Input: part model. Units: mm. Frame: model coordinates. A direction names the side the tool comes from. Coordinates: 2 decimals unless noted, no trailing zeros. Loops run counter-clockwise (first coordinate to the right, second up) from the corner with the lowest first, then second, coordinate; pieces in that order, holes last. Notation, with made-up numbers: (72, 79.5) -> (93, 79.5) arc R16 cw to (93, 110.5) -> close; hole circle Ø1 at (28.5, 53.25). An arc over 180 degrees is marked (long way). Answer as a JSON object with one key per item and string values.
Autodesk Inventor part; units mm, degrees
ref_plane "YZ Plane" through (0, 0, 0) normal (1, 0, 0) x (0, 1, 0)
ref_plane "XZ Plane" through (0, 0, 0) normal (0, 1, 0) x (-1, 0, 0)
ref_plane "XY Plane" through (0, 0, 0) normal (0, 0, 1) x (1, 0, 0)
sketch "Sketch1" plane through (0, 0, 0) normal (0, 0, 1) x (1, 0, 0)
  circle A0 centre (0, 0) radius 31.75
  circle A1 centre (0, 0) radius 25.4
  circle A2 centre (0, 0) radius 6.35
  dimension "d0" = 63.5
  dimension "d1" = 50.8
  dimension "d2" = 12.7
extrude "Extrusion1" add sketch "Sketch1" along normal blind 6.35 contours A0
extrude "Extrusion2" add sketch "Sketch1" along normal blind 6.35 contours A1
extrude "Extrusion3" add sketch "Sketch1" against normal blind 19.05 contours A1
properties part number "2.5ingear proxy"
1. Pin query (flat end, axial travel): P1, Ø1.5, axis at y = -15.5, z = -12, coming from the +X side; P2, Ø1, axis at x = -3.5, z = -1, coming from the +Y side; P3, Ø12, axis at y = 6.5, z = -9, coming from the -X side. Return the tip coordinate at first contact, or that it passes through.
Reply:
{"P1": "stops at x = 20.68", "P2": "stops at y = 25.22", "P3": "stops at x = -25.4"}
2. Section query D-D (x = 13). Return loops of the section in (y, z), plus the area to 3 significant figures.
Reply:
{"outline": "(-28.97, 0) -> (-21.82, 0) -> (-21.82, -19.05) -> (21.82, -19.05) -> (21.82, 0) -> (28.97, 0) -> (28.97, 6.35) -> (-28.97, 6.35) -> close", "area": "1,200 mm2"}
3. Section query A-A (x = 0). Return loops of the section in (y, z).
Reply:
{"outline": "(-31.75, 0) -> (-25.4, 0) -> (-25.4, -19.05) -> (-6.35, -19.05) -> (-6.35, 6.35) -> (-31.75, 6.35) -> close; (6.35, -19.05) -> (25.4, -19.05) -> (25.4, 0) -> (31.75, 0) -> (31.75, 6.35) -> (6.35, 6.35) -> close"}
4. Access query for faces 1 (the face through (-14.3, 21.3, 0)), 2 (the face through (7, 0, 6.35)). Directions: +Z, -Z, +X, -X, +Y, -Y. A direction counts if a zero-diameter tool reaches every point of the face in a straight line with its end or side. Return the directions, or none.
Reply:
{"face 1": "-Z", "face 2": "+Z, +X, -X, +Y, -Y"}
5. Section query C-C (y = 22). Return loops of the section in (x, z).
Reply:
{"outline": "(-22.89, 0) -> (-12.69, 0) -> (-12.69, -19.05) -> (12.69, -19.05) -> (12.69, 0) -> (22.89, 0) -> (22.89, 6.35) -> (-22.89, 6.35) -> close"}
6. Mould query, pull axis Y, two halves, no side actions, for faces 3 (the face through (-5.506, -24.796, -9.392)), 4 (the face through (-1.38, 6.2, -6.53)), 5 (the face through (5, -5, -19.05)). Classes: pulls with the +Y half, pulls with the -Y half, needs draft (parallel to the pull), parting line crosses it, or undercut.
Reply:
{"face 3": "parting line crosses it", "face 4": "undercut", "face 5": "needs draft"}
7. Line query: line 1 along Y through (x, z) = (0, -8.5); line 2 along Z through (x, y) = (26.5, 2); line 3 along Y through (x, z) = (15, -15.5). Output: solid intervals per line, ascending.
Reply:
{"line 1": "y = -25.4 to -6.35, 6.35 to 25.4", "line 2": "z = 0 to 6.35", "line 3": "y = -20.5 to 20.5"}
